Source: three-view drawing plus pictorial views. Frame: mm from the lowest corner of the part. A direction names the side the tool comes from. Give positions to 0.01 mm unless a question says otherwise; leave off trailing zeros. Write each loop counter-clockwise with the first axis right and the second up, starting at its lowest first coordinate (ties: lowest second). Pieces come first, ordered by that corner, then holes. Notation, with made-up numbers: M 65,-26 L 87,-26 A21 cw 87,-17 Z; hole C 48,5 d11. An arc over 180 degrees is marked long. One line per question, with ' | ' between items.
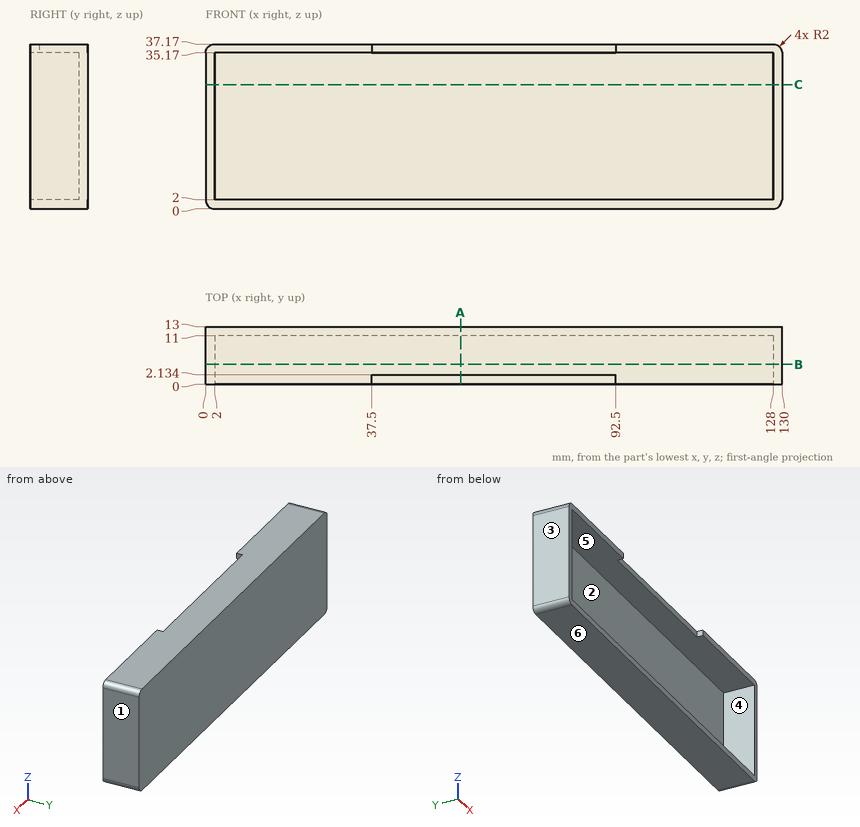
(1) Cut plane B-B, the plane y = 4.5. Return loops of the section in (x, z).
Working result:
outline: M 0,2 A2 ccw 2,0 L 128,0 A2 ccw 130,2 L 130,35.17 A2 ccw 128,37.17 L 2,37.17 A2 ccw 0,35.17 Z; hole M 2,2 L 128,2 L 128,35.17 L 2,35.17 Z
(2) Cut plane C-C, the plane z = 28. Return loops of the section in (x, y).
Working result:
outline: M 0,0 L 2,0 L 2,11 L 128,11 L 128,0 L 130,0 L 130,13 L 0,13 Z
(3) Set-up query: the marked faces 1 and 2. Return all of +Z, -Z, +X, -X, +Y, -Y with unobstructed straight access to the full face (end or side cutting, diameter ignored); none if empty.
Working result:
face 1: +Z, -Z, +X, +Y, -Y | face 2: -Y
(4) Cut plane A-A, the plane x = 57.5. Return loops of the section in (y, z), then the cut area to 3 significant figures.
Working result:
outline: M 0,0 L 13,0 L 13,37.17 L 2.13,37.17 L 2.13,35.17 L 11,35.17 L 11,2 L 0,2 Z | area: 114 mm^2
(5) Material intervals for L1, parallel to Z at x = 70, y = 5.75; L2, parallel to X at y = 3, z = 30.5; L3, parallel to Y at x = 51, z = 28, sorted ascending. Write a range as [from, to].
Working result:
L1: z = [0, 2], [35.17, 37.17] | L2: x = [0, 2], [128, 130] | L3: y = [11, 13]
(6) First-contact query: P1, Ø1.6, axis at y = 1, z = 36.5, coming from the -X side; P2, Ø1.5, axis at x = 57, z = 23, coming from the -Y side; P3, Ø1.6, axis at x = 68.5, z = 36.5, coming from the -Y side. Flat tips, straight axial feed; report the tip coordinate or a pass-through.
Working result:
P1: stops at x = 0.07 | P2: stops at y = 11 | P3: stops at y = 2.13
(7) Draft query along X for the marked faces 3, 4, 5 and 6. Return one class per face: released by +X, released by -X, zero draft, split by the parting line, or undercut.
Working result:
face 3: released by -X | face 4: undercut | face 5: undercut | face 6: zero draft
